CAD build for the part. Positions are in the model's coordinates, mm. A direction names the side the tool comes from. Give positions to 0.01 mm unless a question says otherwise; leave off trailing zeros. Loops run counter-clockwise (first coordinate to the right, second up) from the corner with the lowest first, then second, coordinate; pieces in that order, holes last. Notation, with made-up numbers: (-39, 9.5) -> (-13, 9.5) arc R17 ccw to (-13, 30.5) -> close; hole circle Ø3 at (-18.5, 74). An arc over 180 degrees is marked (long way). Use one line per item in the form item = value.
```python
from build123d import *

# Parameters (mm, degrees)
F1_DEPTH = 5
F2_R     = 10
F3_SIZE  = 1


with BuildPart() as f1:
    # F0 (on Top) → F1 (new body)
    with BuildSketch(Plane.XY):
        Polygon((0, 40), (0, 0), (55, 0), (60, 25), (65, 25), (65, 0), (80, 0), (80, 40), align=None)
    extrude(amount=F1_DEPTH)

    # F2
    f2_edges = [f1.edges().sort_by_distance(p)[0] for p in [
        (80, 0, 2.5),
        (80, 40, 2.5),
        (0, 40, 2.5),
        (0, 0, 2.5),
    ]]
    fillet(f2_edges, radius=F2_R)

    # F3
    f3_edges = [f1.edges().sort_by_distance(p)[0] for p in [
        (77.071068, 2.928932, 5),
        (77.071068, 2.928932, 0),
    ]]
    chamfer(f3_edges, length=F3_SIZE)


solid = f1.part
```
1. Mould opens along X. For faces 3 (the conical face through (3.442, 3.585, 4.826)), 4 (the flat face through (32, 0, 2)), 5 (the flat face through (65, 13, 2)) say: pulls with the +X half, pulls with the -X half, needs draft (parallel to the pull), parting line crosses it, or undercut.
Result sheet:
face_3 = pulls with the -X half
face_4 = needs draft
face_5 = undercut
2. Tool access for faces 1 (the flat face through (57.465, 12.325, 2.465)), 2 (the conical face through (76.558, 36.415, 0.174)): list every direction of +Z, -Z, +X, -X, +Y, -Y with a clear straight run to the whole face (end or side of a thin tool).
Result sheet:
face_1 = +Z, -Z, -Y
face_2 = -Z, +X, +Y
3. Cut at A-A, the plane y = 11.5. Write the cut outline in (x, z), then the cut area to 4 significant figures.
Result sheet:
outline = (0, 1) -> (1, 0) -> (57.3, 0) -> (57.3, 5) -> (1, 5) -> (0, 4) -> close; (65, 0) -> (79, 0) -> (80, 1) -> (80, 4) -> (79, 5) -> (65, 5) -> close
area = 359.5 mm^2
4. Drop a flat-ended pin along its axis: P1, Ø2.5, axis at x = 62.5, z = 1.5, coming from the -Y side. Give the stop position or say it passes through.
Result sheet:
P1 = 25
5. Cut at B-B, the plane y = 21. Write the cut outline in (x, z).
Result sheet:
outline = (0, 1) -> (1, 0) -> (59.2, 0) -> (59.2, 5) -> (1, 5) -> (0, 4) -> close; (65, 0) -> (79, 0) -> (80, 1) -> (80, 4) -> (79, 5) -> (65, 5) -> close
6. Drill centre lines: line 1 (X direction, y = 21, z = 3); line 2 (X direction, y = 8, z = 4.05); line 3 (X direction, y = 38, z = 0.75). Where is each one in solid material? Low to high.
Result sheet:
line_1 = 0 to 59.2, 65 to 80
line_2 = 0.25 to 56.6, 65 to 79.75
line_3 = 4.43 to 75.57
7. Cut at C-C, the plane z = 2.9. Write the cut outline in (x, y), then the cut area to 3 significant figures.
Result sheet:
outline = (0, 10) arc R10 ccw to (10, 0) -> (55, 0) -> (60, 25) -> (65, 25) -> (65, 0) -> (70, 0) arc R10 ccw to (80, 10) -> (80, 30) arc R10 ccw to (70, 40) -> (10, 40) arc R10 ccw to (0, 30) -> close
area = 2,930 mm^2
